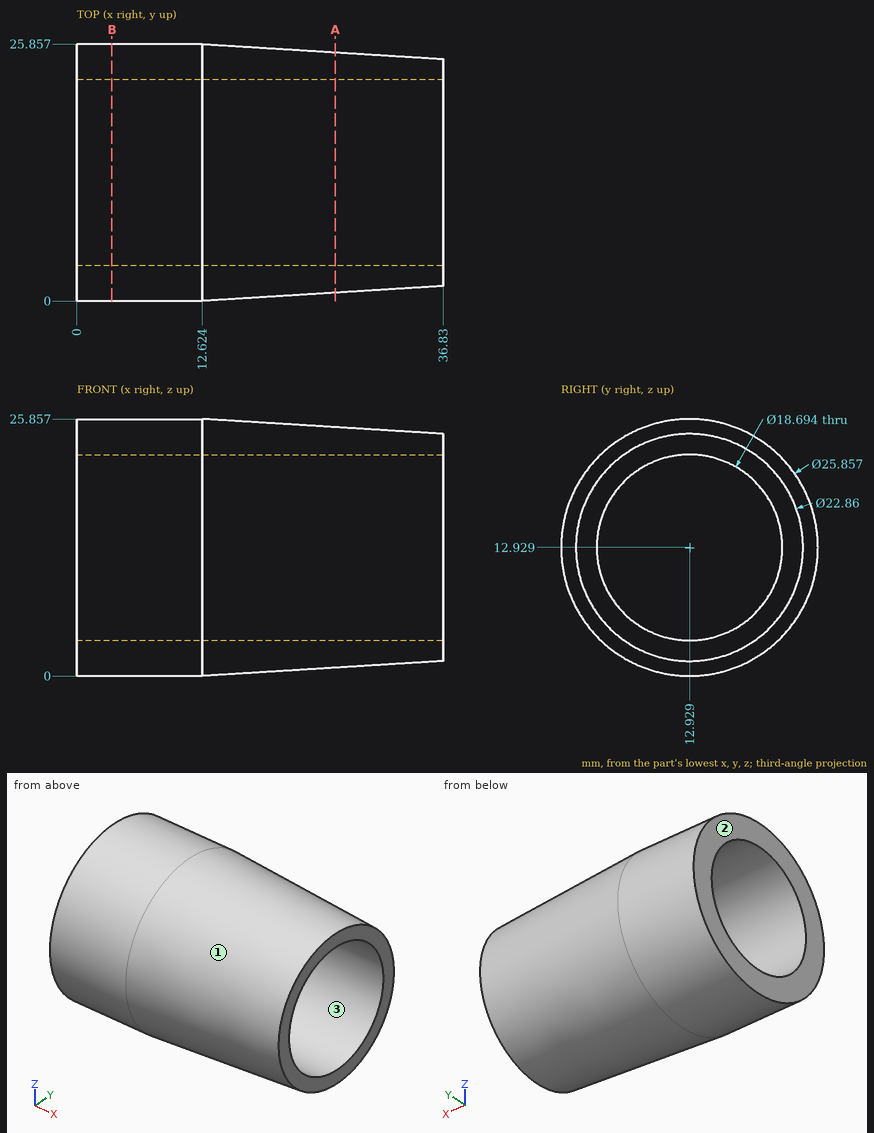
Input: dimensioned drawing with shaded views. Units: mm. Origin: part minimum x, y, z. Coordinates: 2 decimals unless noted, no trailing zeros. Write each loop counter-clockwise with the first axis right and the second up, starting at its lowest first coordinate (ties: lowest second). Pieces come first, ordered by that corner, then holes. Notation, with made-up numbers: M 53.5,30 L 61.5,30 A30 cw 61.5,56 Z; hole C 71.5,80 d4. An arc over 180 degrees is marked long. Use one line per item in the form item = value.
Q1. Draft query along Z for the marked faces 1, 2 and 3. Return one class per face: released by +Z, released by -Z, zero draft, split by the parting line, or undercut.
Answer below:
face_1 = split by the parting line
face_2 = zero draft
face_3 = undercut
Q2. Material intervals for probe 1 along Z at (x, y) = (4.5, 12.5); probe 2 along Z at (x, y) = (7.5, 13) (1 decimal); probe 3 along Y at (x, z) = (6.5, 11.75) (1 decimal), sorted ascending. Write a range as from..to.
Answer below:
probe_1 = 0.01..3.59, 22.27..25.85
probe_2 = 0..3.6, 22.3..25.9
probe_3 = 0.1..3.7, 22.2..25.8
Q3. Section A-A (x = 26). Return loops of the section in (y, z) (1 decimal).
Answer below:
outline = C 12.9,12.9 d24.2; hole C 12.9,12.9 d18.7
Q4. First-contact query: pin 1 (10 mm diameter, centred on x = 18.5, z = 15.5, fed in from -Y); pin 2 (12 mm diameter, centred on x = 8.5, y = 4.5, fed in from -Z); pin 3 (8 mm diameter, centred on x = 26.5, y = 13.5, fed in from -Z). Flat tips, straight axial feed; report the tip coordinate or a pass-through.
Answer below:
pin_1 = 0.09
pin_2 = 0.23
pin_3 = 0.61
Q5. Section B-B (x = 3.5). Return loops of the section in (y, z) (1 decimal).
Answer below:
outline = C 12.9,12.9 d25.9; hole C 12.9,12.9 d18.7
